The listing builds one solid part. Answer for the finished solid, in the listing's coordinates (mm). A direction names the side the tool comes from. Give positions to 0.01 mm unless a question says otherwise; leave off trailing zeros. Write each loop counter-clockwise with the first axis right and the second up, starting at its lowest first coordinate (ties: lowest second). Pieces come first, ordered by that corner, then holes. Notation, with made-up numbers: (49.25, 30.5) - (78.25, 30.5) arc R36 cw to (78.25, 65.5) - close; hole circle Ø6 at (30, 63). An arc over 180 degrees is marked (long way). One line per question, with ' | ' between items. Start each with the question number.
1. Given P1, Ø4, axis at x = 168.5, y = 9.5, coming from the -Z side; P2, Ø8, axis at x = 94.97, y = 44.77, coming from the +Z side, each flat-ended and moving along its own axis, determine where each tip first touches the part or whether it passes through.
2. Find the intervals of material crossed by L1, parallel to X at y = -55, z = 3.5; L2, parallel to Y at x = 209.5, z = 27; L3, parallel to X at y = -49, z = 29, in increasing order. Write a range as from..to.
3. For faces 1 (the face through (240.555, 45.761, 1.972)), 2 (the face through (162, -1, 4)), determine the directions among +Z, -Z, +X, -X, +Y, -Y from which every point of the face is accessible in a straight line to the end or side of a thin tool.
4. A cutting plane is placed at A-A (z = 18.5). Determine the outline of the cut face in (x, y).
5. A cutting plane is placed at B-B (y = -31.5). Determine the outline of the cut face in (x, z), then the cut area to 3 significant figures.
6. The mould has two halves that part along X. Classify faces 3 (the face through (259.442, -3, 16)), 4 (the face through (92.374, -48.503, 1.972)), 5 (the face through (162, -1, 0)): +X half, -X half, draft (parallel to the pull), parting line (faces both ways), or undercut.
7. A cutting plane is placed at C-C (x = 199). Determine the outline of the cut face in (y, z).
```python
from build123d import *

# Parameters (mm, degrees)
SKETCH1_W           = 191.709364395
SKETCH1_H           = 142.845926684
SKETCH1_W_2         = 183.709364395
SKETCH1_H_2         = 134.845926684
SKETCH1_R           = 3.5
BOSS_EXTRUDE2_DEPTH = 4
SKETCH1_5_W         = 191.709364395
SKETCH1_5_H         = 142.845926684
SKETCH1_5_W_2       = 183.709364395
SKETCH1_5_H_2       = 134.845926684
BOSS_EXTRUDE3_DEPTH = 32


with BuildPart() as part:
    # Sketch1 → Boss-Extrude2 (new body)
    with BuildSketch(Plane.XY):
        with Locations((163.587328245, -1.577036658)):
            Rectangle(SKETCH1_W, SKETCH1_H)
        with Locations((163.587328245, -1.577036658)):
            Rectangle(SKETCH1_W_2, SKETCH1_H_2, mode=Mode.SUBTRACT)
        with Locations((163.587328245, -1.577036658)):
            Rectangle(SKETCH1_W_2, SKETCH1_H_2)
        with Locations((79.183060399, -59.680217036)):
            Circle(SKETCH1_R, mode=Mode.SUBTRACT)
        with Locations((95.871017698, -48.656965194)):
            Circle(SKETCH1_R, mode=Mode.SUBTRACT)
        with Locations((242.235781203, -54.69781901)):
            Circle(SKETCH1_R, mode=Mode.SUBTRACT)
        with Locations((225.662040668, -43.503573852)):
            Circle(SKETCH1_R, mode=Mode.SUBTRACT)
        with Locations((237.21688879, 44.709233314)):
            Circle(SKETCH1_R, mode=Mode.SUBTRACT)
        with Locations((220.528931491, 33.685981472)):
            Circle(SKETCH1_R, mode=Mode.SUBTRACT)
        with Locations((111.546962379, 33.572096538)):
            Circle(SKETCH1_R, mode=Mode.SUBTRACT)
        with Locations((94.973221843, 44.766341696)):
            Circle(SKETCH1_R, mode=Mode.SUBTRACT)
    extrude(amount=BOSS_EXTRUDE2_DEPTH)

    # Sketch1_5 → Boss-Extrude3 (add)
    with BuildSketch(Plane.XY):
        with Locations((163.587328245, -1.577036658)):
            Rectangle(SKETCH1_5_W, SKETCH1_5_H)
        with Locations((163.587328245, -1.577036658)):
            Rectangle(SKETCH1_5_W_2, SKETCH1_5_H_2, mode=Mode.SUBTRACT)
    extrude(amount=BOSS_EXTRUDE3_DEPTH)


solid = part.part
```
Determined:
1) P1: z = 0 | P2: z = 4
2) L1: 67.73..238.75, 245.72..259.44 | L2: -73..-69, 65.85..69.85 | L3: 67.73..71.73, 255.44..259.44
3) face 1: +Z, -Z | face 2: +Z
4) outline: (67.73, -73) - (259.44, -73) - (259.44, 69.85) - (67.73, 69.85) - close; hole (71.73, -69) - (255.44, -69) - (255.44, 65.85) - (71.73, 65.85) - close
5) outline: (67.73, 0) - (259.44, 0) - (259.44, 32) - (255.44, 32) - (255.44, 4) - (71.73, 4) - (71.73, 32) - (67.73, 32) - close | area: 991 mm2
6) face 3: +X half | face 4: undercut | face 5: draft
7) outline: (-73, 0) - (69.85, 0) - (69.85, 32) - (65.85, 32) - (65.85, 4) - (-69, 4) - (-69, 32) - (-73, 32) - close
